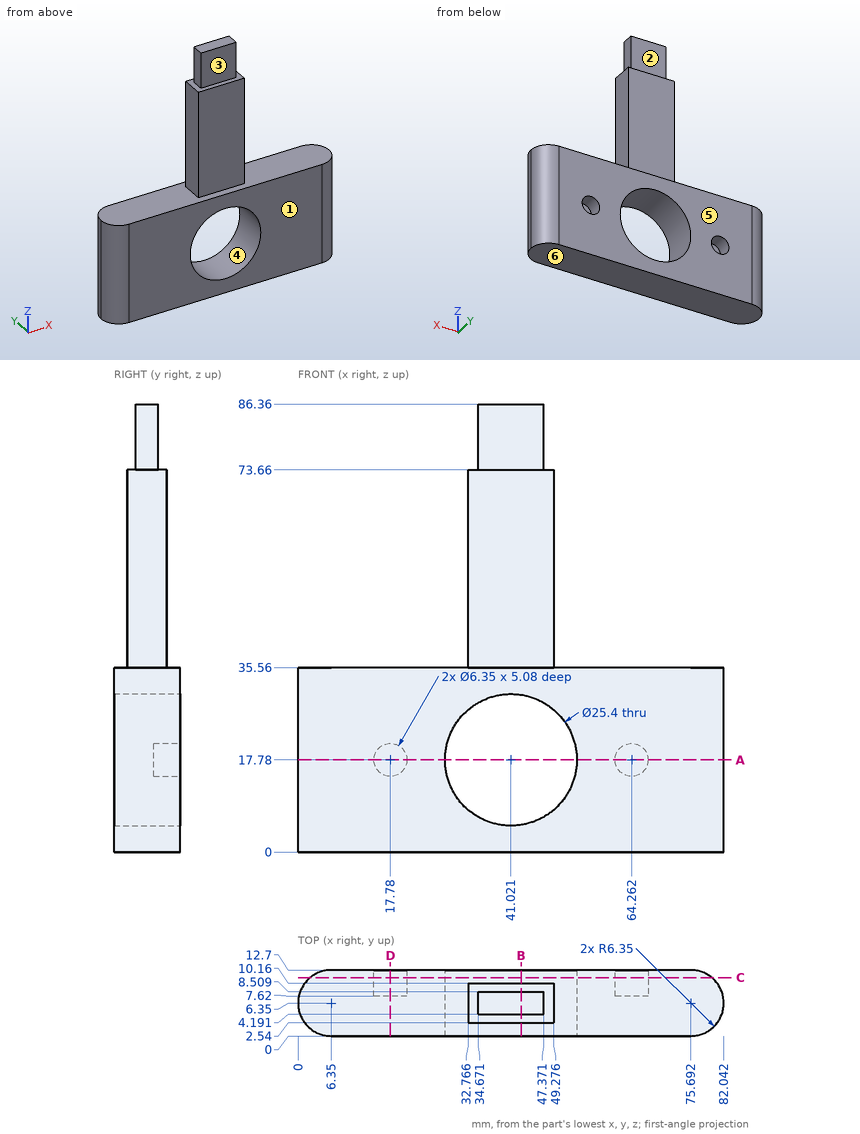
The figure shows three views and two pictorial views of one solid part (mm, origin at its lowest corner). Answer the questions. A direction names the side the tool comes from. Round coordinates to 2 decimals unless told otherwise and drop trailing zeros. Write each loop counter-clockwise with the first axis right and the second up, starting at its lowest first coordinate (ties: lowest second). Pieces come first, ordered by that corner, then holes. Notation, with made-up numbers: M -19,32.5 L -3,32.5 A26 cw -3,60.5 Z; hole C 64,-39 d8. An arc over 180 degrees is marked long. Use a Markdown table: item, result.
1) Straight lines are drawn through the part: line 1 along X through (y, z) = (10.65, 17.78) (3 decimals); line 2 along X through (y, z) = (10.7, 17.78) (3 decimals); line 3 along Y through (x, z) = (45, 47). For each, find the intervals that lie inside material, in ascending order. Write a range as [from, to].
Answers follow:
| item | result |
|---|---|
| line 1 | x = [1.677, 14.605], [20.955, 28.321], [53.721, 61.087], [67.437, 80.365] |
| line 2 | x = [1.724, 14.605], [20.955, 28.321], [53.721, 61.087], [67.437, 80.318] |
| line 3 | y = [2.54, 10.16] |
2) The part is cut by section B-B (x = 43). Write down the section's boundary in (y, z).
Answers follow:
| item | result |
|---|---|
| outline | M 0,0 L 12.7,0 L 12.7,5.24 L 0,5.24 Z; M 0,30.32 L 12.7,30.32 L 12.7,35.56 L 10.16,35.56 L 10.16,73.66 L 8.51,73.66 L 8.51,86.36 L 4.19,86.36 L 4.19,73.66 L 2.54,73.66 L 2.54,35.56 L 0,35.56 Z |
3) The part is cut by section A-A (z = 17.78). Write down the section's boundary in (x, y) (3 decimals), plus the area to 3 significant figures.
Answers follow:
| item | result |
|---|---|
| outline | M 6.35,0 L 28.321,0 L 28.321,12.7 L 20.955,12.7 L 20.955,7.62 L 14.605,7.62 L 14.605,12.7 L 6.35,12.7 A6.35 ccw Z; M 53.721,0 L 75.692,0 A6.35 ccw 75.692,12.7 L 67.437,12.7 L 67.437,7.62 L 61.087,7.62 L 61.087,12.7 L 53.721,12.7 Z |
| area | 620 mm2 |
4) The part is cut by section D-D (x = 17.78). Write down the section's boundary in (y, z) (3 decimals).
Answers follow:
| item | result |
|---|---|
| outline | M 0,0 L 12.7,0 L 12.7,14.605 L 7.62,14.605 L 7.62,20.955 L 12.7,20.955 L 12.7,35.56 L 0,35.56 Z |
5) The part is cut by section C-C (y = 11.25). Write down the section's boundary in (x, z) (3 decimals), plus the area to 3 significant figures.
Answers follow:
| item | result |
|---|---|
| outline | M 2.311,0 L 79.731,0 L 79.731,35.56 L 2.311,35.56 Z; hole C 17.78,17.78 d6.35; hole C 41.021,17.78 d25.4; hole C 64.262,17.78 d6.35 |
| area | 2,180 mm2 |
6) A tool of negligible diameter and unlimited length cuts with its end or side. For the marked faces 1, 2 and 3, from which of +Z, -Z, +X, -X, +Y, -Y can it reach the whole face along a straight path? Write none if from no direction.
Answers follow:
| item | result |
|---|---|
| face 1 | +Z, -Z, +X, -X, -Y |
| face 2 | +Z, +X, -X, +Y |
| face 3 | +Z, +X, -X, -Y |
7) Flat-ended cylindrical pins translate along their axes: pin 1 (6.5 mm diameter, centred on x = 39, z = 81.5, fed in from +Y); pin 2 (2 mm diameter, centred on y = 5.5, z = 81, fed in from -X); pin 3 (3 mm diameter, centred on y = 4, z = 50.5, fed in from -X). Find the tip coordinate at first contact, or state that the pin passes through.
Answers follow:
| item | result |
|---|---|
| pin 1 | stops at y = 8.51 |
| pin 2 | stops at x = 34.67 |
| pin 3 | stops at x = 32.77 |
8) For a pull along Z with two mould halves and no side action, classify the marked faces 4, 5 and 6 as pulls with the +Z half, pulls with the -Z half, needs draft (parallel to the pull), parting line crosses it, or undercut.
Answers follow:
| item | result |
|---|---|
| face 4 | undercut |
| face 5 | needs draft |
| face 6 | pulls with the -Z half |
